Can you work these out from the model? Positions are in its coordinate system, mm. Face numbers are marked on the shaded views. A direction names the side the tool comes from. Coordinates: 2 decimals unless noted, no trailing zeros. Write each loop counter-clockwise with the first axis right and the second up, starting at its lowest first coordinate (ties: lowest second). Pieces come first, ordered by that corner, then holes. Notation, with made-up numbers: (-8, 74) -> (6, 74) arc R7 cw to (6, 85) -> close; hole circle Ø6 at (55.25, 34.25). An arc over 180 degrees is marked (long way). Use one line per item in the form item = value.
```python
from build123d import *

# Parameters (mm, degrees)
SKETCH_W        = 29
SKETCH_H        = 40
PAD_DEPTH       = 8
CHAMFER_SIZE    = 4
CHAMFER001_SIZE = 1
SKETCH001_W     = 20.25
SKETCH001_H     = 20
POCKET_DEPTH    = 15
POCKET001_DEPTH = 6
SKETCH003_W     = 17.593698
SKETCH003_H     = 25.266384
POCKET002_DEPTH = 5
SKETCH004_W     = 4.2
SKETCH004_H     = 5.2
POCKET003_DEPTH = 1.2


with BuildPart() as part:
    # Sketch (on XY_Plane of Origin) → Pad (new body)
    with BuildSketch(Plane.XY):
        Rectangle(SKETCH_W, SKETCH_H)
    extrude(amount=PAD_DEPTH)

    # Chamfer
    chamfer_edges = [part.edges().sort_by_distance(p)[0] for p in [
        (14.5, 20, 4),
        (14.5, -20, 4),
        (-14.5, 20, 4),
        (-14.5, -20, 4),
    ]]
    chamfer(chamfer_edges, length=CHAMFER_SIZE)

    # Chamfer001
    chamfer001_edges = [part.edges().sort_by_distance(p)[0] for p in [
        (0, -20, 0),
        (0, -20, 8),
        (0, 20, 0),
        (0, 20, 8),
    ]]
    chamfer(chamfer001_edges, length=CHAMFER001_SIZE)

    # Sketch001 (on Face8 of Chamfer001) → Pocket (cut)
    with BuildSketch(Plane.XY.offset(8)):
        with Locations((0, -27.031727)):
            Rectangle(SKETCH001_W, SKETCH001_H)
        with Locations((0, 27.031727)):
            Rectangle(SKETCH001_W, SKETCH001_H)
    extrude(amount=-POCKET_DEPTH, mode=Mode.SUBTRACT)

    # Sketch002 (on Face7 of Pocket) → Pocket001 (cut)
    with BuildSketch(Plane.XY.offset(8)):
        with BuildLine():
            ThreePointArc((13.25, 2.75), (0, 16), (-13.25, 2.75))
            Line((-13.25, 2.75), (-13.25, -2.75))
            ThreePointArc((-13.25, -2.75), (0, -16), (13.25, -2.75))
            Line((13.25, 2.75), (13.25, -2.75))
        make_face()
    extrude(amount=-POCKET001_DEPTH, mode=Mode.SUBTRACT)

    # Sketch003 (on Face7 of Pocket001) → Pocket002 (cut)
    with BuildSketch(Plane.XY.offset(8)):
        with Locations((3.091955, 0)):
            Rectangle(SKETCH003_W, SKETCH003_H)
    extrude(amount=-POCKET002_DEPTH, mode=Mode.SUBTRACT)

    # Sketch004 (on Face36 of Pocket002) → Pocket003 (cut)
    with BuildSketch(Plane.XY.offset(2)):
        with Locations((10, -6)):
            Rectangle(SKETCH004_W, SKETCH004_H)
        with Locations((10, 6)):
            Rectangle(SKETCH004_W, SKETCH004_H)
    extrude(amount=-POCKET003_DEPTH, mode=Mode.SUBTRACT)


solid = part.part
```
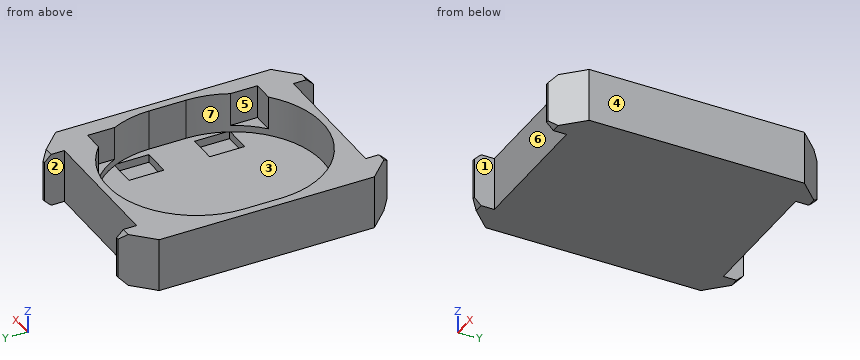
Q1. Thinking about a two-plate mould opening in Y: for the marked faces 4, 5, 6 and 7, which applies, released by +Y, released by -Y, zero draft, split by the parting line, or undercut?
Return value:
face_4 = zero draft
face_5 = undercut
face_6 = released by -Y
face_7 = undercut
Q2. For the marked faces 1, 2 and 3, which set-ups out of +Z, -Z, +X, -X, +Y, -Y let a thin tool reach every point of the face, with its end or its side?
Return value:
face_1 = +Z, -Z, -Y
face_2 = +Z, -Z, +Y
face_3 = +Z
Q3. Suppose I cut it at A-A (z = 6.25). Write out the boundary of the cut face in (x, y) (3 decimals).
Return value:
outline = (-14.5, -16) -> (-10.5, -20) -> (-10.125, -20) -> (-10.125, -17.032) -> (10.125, -17.032) -> (10.125, -20) -> (10.5, -20) -> (14.5, -16) -> (14.5, 16) -> (10.5, 20) -> (10.125, 20) -> (10.125, 17.032) -> (-10.125, 17.032) -> (-10.125, 20) -> (-10.5, 20) -> (-14.5, 16) -> close; hole (-13.25, -2.75) arc R13.25 ccw to (8.825, -12.633) -> (11.889, -12.633) -> (11.889, -8.6) arc R13.25 ccw to (13.25, -2.75) -> (13.25, 2.75) arc R13.25 ccw to (11.889, 8.6) -> (11.889, 12.633) -> (8.825, 12.633) arc R13.25 ccw to (-13.25, 2.75) -> close
Q4. If I drill on line 1 (Y direction, x = 9.25, z = 1.5); line 2 (X direction, y = -1, z = 4); line 3 (Z direction, x = -7, y = -10), over which ranges is the centre line in solid material (lowest first)? Write a range as from..to.
Return value:
line_1 = -17.03..-8.6, -3.4..3.4, 8.6..17.03
line_2 = -14.5..-13.25, 13.25..14.5
line_3 = 0..2
Q5. Suppose I cut it at C-C (y = -1.5). Write out the boundary of the cut face in (x, z), then the cut area to 3 significant figures.
Return value:
outline = (-14.5, 0) -> (14.5, 0) -> (14.5, 8) -> (13.25, 8) -> (13.25, 2) -> (-13.25, 2) -> (-13.25, 8) -> (-14.5, 8) -> close
area = 73.0 mm2
Q6. Suppose I cut it at D-D (y = 5). Write out the boundary of the cut face in (x, z).
Return value:
outline = (-14.5, 0) -> (14.5, 0) -> (14.5, 8) -> (13.06, 8) -> (13.06, 2) -> (12.1, 2) -> (12.1, 0.8) -> (7.9, 0.8) -> (7.9, 2) -> (-13.06, 2) -> (-13.06, 8) -> (-14.5, 8) -> close
Q7. Suppose I cut it at B-B (x = 0). Write out the boundary of the cut face in (y, z), then the cut area to 3 significant figures.
Return value:
outline = (-17.03, 0) -> (17.03, 0) -> (17.03, 8) -> (16, 8) -> (16, 2) -> (-16, 2) -> (-16, 8) -> (-17.03, 8) -> close
area = 80.5 mm2
Q8. Will these pins go through, and if not, where does the flat tip stop? pin 1 (2 mm diameter, centred on x = -4, z = 5, fed in from -Y); pin 2 (2 mm diameter, centred on x = -6, y = 13, fed in from +Z); pin 3 (2.5 mm diameter, centred on y = 18, z = 5, fed in from -X).
Return value:
pin_1 = -17.03
pin_2 = 2
pin_3 = -13.75
